from build123d import *

# Parameters (mm, degrees)
BOSS_EXTRU_1_DEPTH      = 6.35
ESQUISSE2_W             = 20
ESQUISSE2_H             = 6.35
ESQUISSE2_W_2           = 6.35
ESQUISSE2_H_2           = 20
ENL_V_MAT_EXTRU_1_DEPTH = 157.601902923
CONG_1_R                = 6
CONG_2_R                = 2
ENL_V_MAT_EXTRU_2_DEPTH = 157.601902923
CONG_4_R                = 3


with BuildPart() as part:
    # Esquisse1 → Boss.-Extru.1 (new body)
    with BuildSketch(Plane(origin=(0, 0, 0), x_dir=(0, 0, -1), z_dir=(1, 0, 0))):
        Polygon((-42.072853481, 0), (42.072853481, 0), (42.072853481, 84.949747468), (30.759144982, 96.263455967), (26.516504294, 92.02081528), (33.587572106, 84.949747468), (28.637824638, 80), (-42.072853481, 150.710678119), align=None)
    extrude(amount=BOSS_EXTRU_1_DEPTH)

    # Esquisse2 → Enlèv. mat.-Extru.1 (cut, through all)
    with BuildSketch(Plane(origin=(6.35, 0, 0), x_dir=(0, 0, -1), z_dir=(1, 0, 0))):
        with Locations((0, 3.175)):
            Rectangle(ESQUISSE2_W, ESQUISSE2_H)
        with Locations((0, 49.525)):
            Rectangle(ESQUISSE2_W, ESQUISSE2_H)
        with Locations((38.897853481, 26.35)):
            Rectangle(ESQUISSE2_W_2, ESQUISSE2_H_2)
    extrude(amount=-ENL_V_MAT_EXTRU_1_DEPTH, mode=Mode.SUBTRACT)

    # Congé1
    cong_1_edges = [part.edges().sort_by_distance(p)[0] for p in [
        (3.175, 84.949747468, -42.072853481),
    ]]
    fillet(cong_1_edges, radius=CONG_1_R)

    # Congé2
    cong_2_edges = [part.edges().sort_by_distance(p)[0] for p in [
        (3.175, 92.02081528, -26.516504294),
        (3.175, 96.263455967, -30.759144982),
    ]]
    fillet(cong_2_edges, radius=CONG_2_R)

    # Esquisse4 → Enlèv. mat.-Extru.2 (cut, through all)
    with BuildSketch(Plane(origin=(6.35, 0, 0), x_dir=(0, 0, -1), z_dir=(1, 0, 0))):
        Polygon((24.624116139, 72.7), (-34.072853481, 72.7), (-34.072853481, 131.39696962), align=None)
    extrude(amount=-ENL_V_MAT_EXTRU_2_DEPTH, mode=Mode.SUBTRACT)

    # Congé4
    cong_4_edges = [part.edges().sort_by_distance(p)[0] for p in [
        (3.175, 150.710678119, 42.072853481),
        (3.175, 131.39696962, 34.072853481),
        (3.175, 72.7, -24.624116139),
        (3.175, 72.7, 34.072853481),
    ]]
    fillet(cong_4_edges, radius=CONG_4_R)


solid = part.part
Check sheet for the modelled part. Datum: model origin and axes. Units: mm. A direction names the side the tool comes from. Give positions to 0.01 mm unless a question says otherwise; leave off trailing zeros. Write each loop counter-clockwise with the first axis right and the second up, starting at its lowest first coordinate (ties: lowest second). Pieces come first, ordered by that corner, then holes. Notation, with made-up numbers: (85, 49.5) -> (138, 49.5) arc R26 ccw to (138, 63.5) -> close; hole circle Ø4 at (40.25, 52.25). An arc over 180 degrees is marked (long way). Write item = value, one per line.
Item 1: Sectioned sample at C-C on z = -15.5. Record the boundary of the cut face in (x, y), and give its area (3 significant figures).
Output:
outline = (0, 0) -> (6.35, 0) -> (6.35, 72.7) -> (0, 72.7) -> close; (0, 81.82) -> (6.35, 81.82) -> (6.35, 93.14) -> (0, 93.14) -> close
area = 533 mm^2
Item 2: Tool access check on faces 1 (the flat face through (3, 36.35, -39)), 2 (the cylindrical face through (3.2, 84.8, -41.6)), 3 (the flat face through (3, 49, -10)), 4 (the flat face through (3, 3, -10)), 5 (the flat face through (3, 8, -42.073)). Record the directions out of +Z, -Z, +X, -X, +Y, -Y that give a thin tool (end or side, any length) a straight path to the whole face; none if there is none.
Output:
face_1 = -Z, +X, -X
face_2 = -Z, +X, -X, +Y
face_3 = +X, -X
face_4 = +X, -X, -Y
face_5 = -Z, +X, -X, +Y, -Y
Item 3: Gauge pin test, flat ends, axial feed: pin 1 (2 mm diameter, centred on x = 4.5, z = 1, fed in from -Y); pin 2 (1.9 mm diameter, centred on x = 4.5, z = -2, fed in from +Y); pin 3 (3 mm diameter, centred on x = 2, z = -38, fed in from +Y). Record the tip position at first contact, or that the pin passes through.
Output:
pin_1 = 6.35
pin_2 = 107.59
pin_3 = 90.52
Item 4: Release check for a two-part mould opening along Z. For faces 6 (the cylindrical face through (3.219, 146.258, 40.175)), 7 (the flat face through (3, 26, -35.723)), 8 (the cylindrical face through (3.219, 92.043, -27.345)) record: +Z half, -Z half, draft (parallel to the pull), parting line (faces both ways), or undercut.
Output:
face_6 = parting line
face_7 = -Z half
face_8 = undercut
Item 5: Sectioned sample at B-B on y = 108.5. Record the boundary of the cut face in (x, z).
Output:
outline = (0, -0.14) -> (6.35, -0.14) -> (6.35, 11.18) -> (0, 11.18) -> close; (0, 34.07) -> (6.35, 34.07) -> (6.35, 42.07) -> (0, 42.07) -> close
Item 6: Sectioned sample at A-A on x = 3. Count the separate pieces of the cut face and the enclosed holes in it, and give its area (3 significant figures).
Output:
separate_pieces = 1
enclosed_holes = 2
area = 7,270 mm^2
Item 7: Scan lines: probe 1 along Z at (x, y) = (4.25, 50); probe 2 along Z at (x, y) = (1.75, 89); probe 3 along Y at (x, z) = (3.25, 2). Record each from-to range of solid material in increasing order. Write a range as from..to.
Output:
probe_1 = -42.07..-10, 10..42.07
probe_2 = -38.02..-29.54, -19.64..-8.32, 34.07..42.07
probe_3 = 6.35..46.35, 52.7..72.7, 99.32..110.64
Item 8: Sectioned sample at D-D on y = 131.5. Record the boundary of the cut face in (x, z).
Output:
outline = (0, 22.86) -> (6.35, 22.86) -> (6.35, 42.07) -> (0, 42.07) -> close
